Could you check a few things on this model? Use its own coordinates, in mm. Face numbers are marked on the shaded views. A direction names the side the tool comes from. Coordinates: 2 decimals unless noted, no trailing zeros. Loops run counter-clockwise (first coordinate to the right, second up) from the corner with the lowest first, then second, coordinate; pieces in that order, holes last. Notation, with made-up numbers: (16, 55) - (54, 55) arc R16 cw to (54, 75) - close; hole circle Ø2 at (-34.5, 47.5). An arc over 180 degrees is marked (long way). Use CSV: the item, a comma, the result in double quotes.
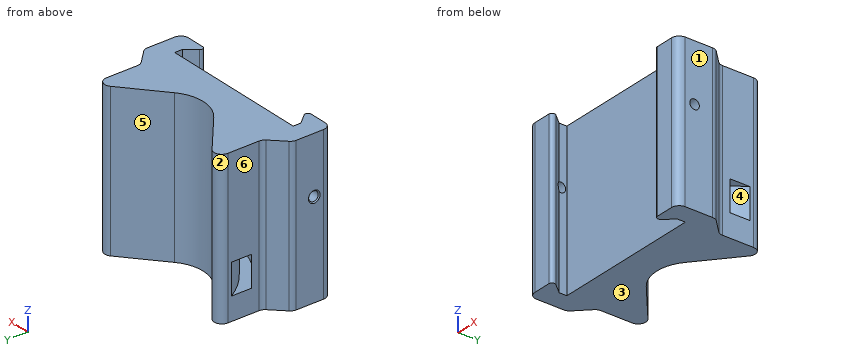
from build123d import *

# Parameters (mm, degrees)
BOSS_EXTRUDE1_DEPTH             = 40
SKETCH2_W                       = 8
SKETCH2_H                       = 3
M3X0_5_TAPPED_HOLE1_D           = 2.5
M3X0_5_TAPPED_HOLE1_CSINK_D     = 3.05
M3X0_5_TAPPED_HOLE1_CSINK_ANGLE = 90


with BuildPart() as part:
    # Sketch1 → Boss-Extrude1 (new body)
    with BuildSketch(Plane.XY):
        with BuildLine():
            Line((6.427876097, 10.393628462), (16.714424781, 19.025067669))
            ThreePointArc((16.714424781, 19.025067669), (18.845236523, 19.305594357), (20, 17.492978783))
            Line((20, 17.492978783), (20, 9.328427125))
            ThreePointArc((20, 9.328427125), (20.152240935, 8.56306026), (20.585786438, 7.914213562))
            Line((20.585786438, 7.914213562), (23.914213562, 4.585786438))
            ThreePointArc((23.914213562, 4.585786438), (24.347759065, 3.93693974), (24.5, 3.171572875))
            Line((24.5, 3.171572875), (24.5, -4))
            ThreePointArc((24.5, -4), (23.914213562, -5.414213562), (22.5, -6))
            Line((22.5, -6), (17.859207012, -6))
            ThreePointArc((17.859207012, -6), (17.134160782, -5.538094609), (17.246371457, -4.685769912))
            Line((17.246371457, -4.685769912), (19.5, -2))
            Line((19.5, -2), (19.5, 0))
            Line((19.5, 0), (-19.5, 0))
            Line((-19.5, 0), (-19.5, -2))
            Line((-19.5, -2), (-17.246371457, -4.685769912))
            ThreePointArc((-17.246371457, -4.685769912), (-17.134160782, -5.538094609), (-17.859207012, -6))
            Line((-17.859207012, -6), (-22.5, -6))
            ThreePointArc((-22.5, -6), (-23.914213562, -5.414213562), (-24.5, -4))
            Line((-24.5, -4), (-24.5, 3.171572875))
            ThreePointArc((-24.5, 3.171572875), (-24.347759065, 3.93693974), (-23.914213562, 4.585786438))
            Line((-23.914213562, 4.585786438), (-20.585786438, 7.914213562))
            ThreePointArc((-20.585786438, 7.914213562), (-20.152240935, 8.56306026), (-20, 9.328427125))
            Line((-20, 9.328427125), (-20, 17.492978783))
            ThreePointArc((-20, 17.492978783), (-18.845236523, 19.305594357), (-16.714424781, 19.025067669))
            Line((-16.714424781, 19.025067669), (-6.427876097, 10.393628462))
            ThreePointArc((-6.427876097, 10.393628462), (0, 8.054072893), (6.427876097, 10.393628462))
        make_face()
    extrude(amount=BOSS_EXTRUDE1_DEPTH)

    # Sketch2 → Cut-Revolve1 (revolve, cut)
    with BuildSketch(Plane(origin=(0, 0, 0), x_dir=(0, 0, -1), z_dir=(1, 0, 0))):
        with Locations((-10, 3.5)):
            Rectangle(SKETCH2_W, SKETCH2_H)
        with Locations((-50, 3.5)):
            Rectangle(SKETCH2_W, SKETCH2_H)
        with Locations((-90, 3.5)):
            Rectangle(SKETCH2_W, SKETCH2_H)
    revolve(axis=Axis((0, 28.054072893, 29.353848425), (0, 0, -1)), mode=Mode.SUBTRACT)

    # M3x0.5 Tapped Hole1 (through all)
    with Locations(Plane.ZY.offset(24.5)):
        with Locations((25, -1.555540573), (75, -1.555540573)):
            CounterSinkHole(M3X0_5_TAPPED_HOLE1_D / 2, M3X0_5_TAPPED_HOLE1_CSINK_D / 2, counter_sink_angle=M3X0_5_TAPPED_HOLE1_CSINK_ANGLE)


solid = part.part
(1) Suppose I cut it at B-B (x = -1). Write out the boundary of the cut face in (y, z), plus the area to 3 significant figures.
Computed:
outline,"(0, 0) - (8.1, 0) - (8.1, 40) - (0, 40) - close; hole (2.02, 6) - (5.02, 6) - (5.02, 14) - (2.02, 14) - close"
area,"300 mm²"
(2) Which directions (+Z, -Z, +X, -X, +Y, -Y) give clear straight access to the entire face, cutting with the end or side of a thin tool? Please do the marked faces 4, 5 and 6.
Computed:
face 4,"none"
face 5,"+Z, -Z, +Y"
face 6,"+Z, -Z, -X, +Y"
(3) Suppose I cut it at D-D (y = 7). Write out the boundary of the cut face in (x, z).
Computed:
outline,"(-21.5, 0) - (21.5, 0) - (21.5, 40) - (-21.5, 40) - close; hole (-15.35, 6) - (-9.39, 6) - (-9.39, 14) - (-15.35, 14) - close; hole (9.39, 6) - (15.35, 6) - (15.35, 14) - (9.39, 14) - close"
(4) Suppose I cut it at A-A (z = 25). State how many separate pieces and enclosed holes the cut face has, plus the area to 3 significant figures.
Computed:
separate pieces,"3"
enclosed holes,"0"
area,"643 mm²"
(5) Please list where these lines run through material, in increasing order: line 1 (Z direction, x = -1, y = 4.75); line 2 (X direction, y = -0.75, z = 18); line 3 (X direction, y = 4, z = 8).
Computed:
line 1,"z = 0 to 6, 14 to 40"
line 2,"x = -24.5 to -19.5, 19.5 to 24.5"
line 3,"x = -24.32 to -10.01, 10.01 to 24.32"
(6) Will these pins go through, and if not, where does the flat tip stop? pin 1 (11.5 mm diameter, centred on x = 9, z = 17.5, fed in from -Y); pin 2 (6 mm diameter, centred on y = 12.5, z = 34, fed in from -X); pin 3 (2 mm diameter, centred on y = -1.56, z = 25, fed in from +X); pin 4 (6.5 mm diameter, centred on y = 12.5, z = 27.5, fed in from +X).
Computed:
pin 1,"stops at y = 0"
pin 2,"stops at x = -20"
pin 3,"passes through"
pin 4,"stops at x = 20"
(7) Suppose I cut it at C-C (y = 12). Write out the boundary of the cut face in (x, z).
Computed:
outline,"(-20, 0) - (-8.34, 0) - (-8.34, 40) - (-20, 40) - (-20, 14) - (-16.55, 14) - (-16.55, 6) - (-20, 6) - close; (8.34, 0) - (20, 0) - (20, 6) - (16.55, 6) - (16.55, 14) - (20, 14) - (20, 40) - (8.34, 40) - close"
(8) Thinking about a two-plate mould opening in X: for the marked faces 1, 2 and 3, which applies, +X half, -X half, draft (parallel to the pull), parting line (faces both ways), or undercut?
Computed:
face 1,"+X half"
face 2,"undercut"
face 3,"draft"
